from build123d import *

# Parameters (mm, degrees)
SKETCH1_W           = 8
SKETCH1_H           = 3.6
BOSS_EXTRUDE1_DEPTH = 4.5
SKETCH2_W           = 3.6
SKETCH2_H           = 3.6
BOSS_EXTRUDE2_DEPTH = 0.7
BOSS_EXTRUDE2_TAPER = 45
SKETCH3_W           = 1.692
SKETCH3_H           = 1.692
BOSS_EXTRUDE3_DEPTH = 2.1
FILLET1_R           = 0.254


with BuildPart() as part:
    # Sketch1 → Boss-Extrude1 (new body)
    with BuildSketch(Plane(origin=(0, 0, 0), x_dir=(1, 0, 0), z_dir=(0, 1, 0))):
        Rectangle(SKETCH1_W, SKETCH1_H)
    extrude(amount=BOSS_EXTRUDE1_DEPTH)

    # Sketch2 → Boss-Extrude2 (add)
    with BuildSketch(Plane(origin=(0, 4.5, 0), x_dir=(1, 0, 0), z_dir=(0, 1, 0))):
        with Locations((2.2, 0)):
            Rectangle(SKETCH2_W, SKETCH2_H)
    extrude(amount=BOSS_EXTRUDE2_DEPTH, taper=BOSS_EXTRUDE2_TAPER)

    # Sketch3 → Boss-Extrude3 (add)
    with BuildSketch(Plane(origin=(0, 5.2, 0), x_dir=(1, 0, 0), z_dir=(0, 1, 0))):
        with Locations((2.2, 0)):
            Rectangle(SKETCH3_W, SKETCH3_H)
    extrude(amount=BOSS_EXTRUDE3_DEPTH)

    # Fillet1
    fillet1_edges = [part.edges().sort_by_distance(p)[0] for p in [
        (2.2, 7.3, 0.846),
        (3.046, 7.3, 0),
        (2.2, 7.3, -0.846),
        (1.354, 7.3, 0),
    ]]
    fillet(fillet1_edges, radius=FILLET1_R)


solid = part.part
Geometry: final body of the model. Coordinates: model frame, mm. A direction names the side the tool comes from. Round coordinates to 2 decimals unless told otherwise and drop trailing zeros. Order: outer loops, then holes, each group sorted by start corner. A loop starts at its lowest first (then second) coordinate and runs counter-clockwise, first axis right, second up. Notation, with made-up numbers: (46.5, -7.5) -> (89.5, -7.5) arc R5 cw to (89.5, -0.5) -> close; hole circle Ø10 at (-3.5, 24.25). An arc over 180 degrees is marked (long way). Put each result on its own line as item: value. Start each with the question number.
Q1. First-contact query: pin 1 (1.9 mm diameter, centred on x = 2, y = 5.5, fed in from -Z); pin 2 (1.8 mm diameter, centred on x = -2.5, z = 0.5, fed in from +Y); pin 3 (1.4 mm diameter, centred on x = 2.5, y = 6.5, fed in from +Z); pin 4 (2 mm diameter, centred on x = -2, y = 5, fed in from +Z). Flat tips, straight axial feed; report the tip coordinate or a pass-through.
Q2. Section B-B on x = -3.25. Return the cut outline in (y, z), and give its area (3 significant figures).
Q3. Section A-A on y = 5.75. Return the cut outline in (x, z).
Q4. Line query: probe 1 along Y at (x, z) = (-0.25, -0.7); probe 2 along Y at (x, z) = (3, 1); probe 3 along X at (y, z) = (6, -0.25). Output: solid intervals per line, ascending.
Q5. Reachability of faces 1 (the flat face through (3.046, 6, 0)), 2 (the flat face through (2, 6, 0.846)), 3 (the flat face through (-2, 4.5, 0)), 4 (the flat face through (2, 6, -0.846)) from +Z, -Z, +X, -X, +Y, -Y: full face, straight path, thin tool, end or side. Return the list, or none.
Ans:
1. pin 1: stops at z = -1.75
1. pin 2: stops at y = 4.5
1. pin 3: stops at z = 0.85
1. pin 4: stops at z = 1.8
2. outline: (0, -1.8) -> (4.5, -1.8) -> (4.5, 1.8) -> (0, 1.8) -> close
2. area: 16.2 mm2
3. outline: (1.35, -0.85) -> (3.05, -0.85) -> (3.05, 0.85) -> (1.35, 0.85) -> close
4. probe 1: y = 0 to 4.5
4. probe 2: y = 0 to 5.2
4. probe 3: x = 1.35 to 3.05
5. face 1: +Z, -Z, +X, +Y
5. face 2: +Z, +X, -X, +Y
5. face 3: +Z, -Z, -X, +Y
5. face 4: -Z, +X, -X, +Y
